Read the model definition and answer for the solid it produces. Units are mm, in the model's axes. A direction names the side the tool comes from. Give positions to 0.01 mm unless a question says otherwise; leave off trailing zeros. Order: outer loops, then holes, each group sorted by start corner. A loop starts at its lowest first (then second) coordinate and runs counter-clockwise, first axis right, second up.
```python
from build123d import *

# Parameters (mm, degrees)
BOSS_EXTRUDE1_DEPTH   = 5
CHAMFER1_SIZE         = 5
BOSS_EXTRUDE5_DEPTH   = 5
CHAMFER2_SIZE         = 2
SKETCH9_R             = 20
CUT_EXTRUDE4_DEPTH    = 5
M6_TAPPED_HOLE1_D     = 5
M4_TAPPED_HOLE1_D     = 3.3
M4_TAPPED_HOLE1_DEPTH = 5
M4_TAPPED_HOLE1_TIP   = 0.991420021


with BuildPart() as part:
    # Sketch1 → Boss-Extrude1 (new body)
    with BuildSketch(Plane(origin=(0, 0, 0), x_dir=(1, 0, 0), z_dir=(0, 1, 0))):
        Polygon((-110, -150), (110, -150), (110, 50), (-102.5, 50), (-110, 50), align=None)
    extrude(amount=BOSS_EXTRUDE1_DEPTH)

    # Chamfer1
    chamfer1_edges = [part.edges().sort_by_distance(p)[0] for p in [
        (110, 2.5, -50),
        (-110, 2.5, -50),
    ]]
    chamfer(chamfer1_edges, length=CHAMFER1_SIZE)

    # Sketch4 → Boss-Extrude5 (add)
    with BuildSketch(Plane.XZ):
        Polygon((95, 135), (0, 135), (-95, 135), (-95, -35), (95, -35), align=None)
        Polygon((-90, 130), (0, 130), (90, 130), (90, -30), (-90, -30), align=None, mode=Mode.SUBTRACT)
    extrude(amount=BOSS_EXTRUDE5_DEPTH)

    # Chamfer2
    chamfer2_edges = [part.edges().sort_by_distance(p)[0] for p in [
        (0, -5, 135),
        (-95, -5, 50),
        (0, -5, -35),
        (95, -5, 50),
    ]]
    chamfer(chamfer2_edges, length=CHAMFER2_SIZE)

    # Sketch9 → Cut-Extrude4 (cut)
    with BuildSketch(Plane(origin=(0, 5, 0), x_dir=(1, 0, 0), z_dir=(0, 1, 0))):
        with Locations(Location((40, -105, 0), (0, 0, 270))):
            Circle(SKETCH9_R)
        with Locations(Location((-40, -105, 0), (0, 0, 270))):
            Circle(SKETCH9_R)
    extrude(amount=-CUT_EXTRUDE4_DEPTH, mode=Mode.SUBTRACT)

    # M6 Tapped Hole1 (through all)
    with Locations(Plane(origin=(0, 5, 0), x_dir=(1, 0, 0), z_dir=(0, 1, 0))):
        with Locations((-102.5, 42.5), (0, 42.5), (102.5, 42.5), (102.5, -50), (-102.5, -50), (-102.5, -142.5), (0, -142.5), (102.5, -142.5)):
            Hole(M6_TAPPED_HOLE1_D / 2)

    # M4 Tapped Hole1
    with Locations(Plane(origin=(0, 5, 0), x_dir=(1, 0, 0), z_dir=(0, 1, 0))):
        with Locations((-59.091883092, -85.908116908), (-20.908116908, -85.908116908), (-20.908116908, -124.091883092), (-59.091883092, -124.091883092), (20.908116908, -85.908116908), (59.091883092, -85.908116908), (59.091883092, -124.091883092), (20.908116908, -124.091883092)):
            Hole(M4_TAPPED_HOLE1_D / 2, depth=M4_TAPPED_HOLE1_DEPTH)
            with Locations((0, 0, -(M4_TAPPED_HOLE1_DEPTH + M4_TAPPED_HOLE1_TIP / 2))):  # 118° drill point
                Cone(0, M4_TAPPED_HOLE1_D / 2, M4_TAPPED_HOLE1_TIP, mode=Mode.SUBTRACT)


solid = part.part
```
1) The part is cut by section B-B on z = 50. Determine the outline of the cut face in (x, y), and give its area (3 significant figures).
Final values:
outline: (-110, 0) - (-105, 0) - (-105, 5) - (-110, 5) - close; (-100, 0) - (-95, 0) - (-95, -3) - (-93, -5) - (-90, -5) - (-90, 0) - (90, 0) - (90, -5) - (93, -5) - (95, -3) - (95, 0) - (100, 0) - (100, 5) - (-100, 5) - close; (105, 0) - (110, 0) - (110, 5) - (105, 5) - close
area: 1,100 mm2
2) Given pin 1 (3.5 mm diameter, centred on y = -1, z = 83, fed in from +X); pin 2 (4 mm diameter, centred on y = -3, z = 55, fed in from +X); pin 3 (8 mm diameter, centred on x = 102.5, z = 50, fed in from -Y), each flat-ended and moving along its own axis, determine where each tip first touches the part or whether it passes through.
Final values:
pin 1: stops at x = 110
pin 2: stops at x = 95
pin 3: stops at y = 0
3) A tool of negligible diameter and unlimited length cuts with its end or side. For faces 5 (the face through (100.115, 2.465, -43.251)), 6 (the face through (-1, 0, 49)), from which of +Z, -Z, +X, -X, +Y, -Y can it reach the whole face along a straight path? Write none if from no direction.
Final values:
face 5: +Y, -Y
face 6: -Y
4) For a pull along Z with two mould halves and no side action, classify faces 1 (the face through (-104.885, 2.465, -43.251)), 2 (the face through (107, 2, -48)), 3 (the face through (-90, -2, 49)), 4 (the face through (110, 2, 54)) as released by +Z, released by -Z, zero draft, split by the parting line, or undercut.
Final values:
face 1: undercut
face 2: released by -Z
face 3: undercut
face 4: zero draft
5) The part is cut by section A-A on x = 102.5. Determine the outline of the cut face in (y, z), and give its area (3 significant figures).
Final values:
outline: (0, -50) - (5, -50) - (5, -45) - (0, -45) - close; (0, -40) - (5, -40) - (5, 47.5) - (0, 47.5) - close; (0, 52.5) - (5, 52.5) - (5, 140) - (0, 140) - close; (0, 145) - (5, 145) - (5, 150) - (0, 150) - close
area: 925 mm2
6) The part is cut by section D-D on z = 4. Determine the outline of the cut face in (x, y).
Final values:
outline: (-110, 0) - (-95, 0) - (-95, -3) - (-93, -5) - (-90, -5) - (-90, 0) - (90, 0) - (90, -5) - (93, -5) - (95, -3) - (95, 0) - (110, 0) - (110, 5) - (-110, 5) - close
7) Consider L1, parallel to X at y = 0.5, z = 50; L2, parallel to X at y = 2, z = 142.5; L3, parallel to Z at x = 0, y = 3.9. Determine where each line is inside the solid, lowest interval first.
Final values:
L1: x = -110 to -105, -100 to 100, 105 to 110
L2: x = -110 to -105, -100 to -2.5, 2.5 to 100, 105 to 110
L3: z = -50 to -45, -40 to 140, 145 to 150
8) The part is cut by section C-C on x = 0. Determine the outline of the cut face in (y, z).
Final values:
outline: (-5, -33) - (-3, -35) - (0, -35) - (0, -40) - (5, -40) - (5, 140) - (0, 140) - (0, 135) - (-3, 135) - (-5, 133) - (-5, 130) - (0, 130) - (0, -30) - (-5, -30) - close; (0, -50) - (5, -50) - (5, -45) - (0, -45) - close; (0, 145) - (5, 145) - (5, 150) - (0, 150) - close
